Autodesk Fusion 360 part; units mm, degrees
sketch "Sketch1" plane through (0, 0, 0) normal (0, 1, 0) x (1, 0, 0)
  line L0 (0, 0) -> (56, 0)
  line L1 (56, 0) -> (56, -65)
  line L2 (56, -65) -> (0, -65)
  line L3 (0, -65) -> (0, 0)
  dimension "d1" = 56
  dimension "d2" = 65
extrude "Extrude1" add sketch "Sketch1" along normal blind 1
sketch "Sketch2" plane through (0, 1, 0) normal (0, 1, 0) x (-1, 0, 0)
  line L0 (0, 65) -> (-56, 65)
  line L1 (-56, 65) -> (-56, 0)
  line L2 (-56, 0) -> (0, 0)
  line L3 (0, 0) -> (0, 65)
  line L4 (-1.5, 7) -> (-5.5, 7)
  line L5 (-5.5, 7) -> (-5.5, 58)
  line L6 (-5.5, 58) -> (-1.5, 58)
  line L7 (-1.5, 58) -> (-1.5, 7)
  dimension "d5" = 4
  dimension "d6" = 51
  dimension "d7" = 7
  dimension "d8" = 7
  dimension "d9" = 1.5
extrude "Extrude2" add sketch "Sketch2" along normal blind 11 contours L4 L5 L6 L7
sketch "Sketch3" plane through (0, 0, 0) normal (0, -1, 0) x (1, 0, 0)
  line L0 (56, 65) -> (0, 65)
  line L1 (0, 65) -> (0, 0)
  line L2 (0, 0) -> (56, 0)
  line L3 (56, 0) -> (56, 65)
  line L4 (1.5, 7) -> (5.5, 7)
  line L5 (5.5, 7) -> (5.5, 58)
  line L6 (5.5, 58) -> (1.5, 58)
  line L7 (1.5, 58) -> (1.5, 7)
extrude "Extrude3" add sketch "Sketch3" along normal blind 14 contours L4 L5 L6 L7
sketch "Sketch4" plane through (0, 1, 0) normal (0, 1, 0) x (-1, 0, 0)
  line L0 (-1.5, 58) -> (-1.5, 7)
  line L1 (-1.5, 7) -> (-5.5, 7)
  line L2 (-5.5, 7) -> (-5.5, 58)
  line L3 (-5.5, 58) -> (-1.5, 58)
  line L4 (0, 65) -> (-56, 65)
  line L5 (-56, 65) -> (-56, 0)
  line L6 (-56, 0) -> (0, 0)
  line L7 (0, 0) -> (0, 65)
  line L8 (-11.1237, 3.0691) -> (-51.1237, 3.0691)
  line L9 (-51.1237, 3.0691) -> (-51.1237, 63.0691)
  line L10 (-51.1237, 63.0691) -> (-11.1237, 63.0691)
  line L11 (-11.1237, 63.0691) -> (-11.1237, 3.0691)
  dimension "d14" = 40
  dimension "d15" = 60
extrude "Extrude4" add sketch "Sketch4" along normal blind 9 contours L8 L9 L10 L11
For this review, take the finished solid that the model builds, in its own axes (mm). A direction names the side the tool comes from. Coordinates: 2 decimals unless noted, no trailing zeros. Write each loop counter-clockwise with the first axis right and the second up, starting at its lowest first coordinate (ties: lowest second). Pieces come first, ordered by that corner, then holes. Notation, with made-up numbers: (-10.75, 86) - (5.25, 86) arc R14 ccw to (5.25, 96) - close; hole circle Ø4 at (11, -35.5). An arc over 180 degrees is marked (long way). Put each result on its own line as item: value.
1. For pin 1 (4.5 mm diameter, centred on x = 40, y = 3.5, fed in from +Z); pin 2 (3.5 mm diameter, centred on y = 6.5, z = 20, fed in from +X); pin 3 (4.5 mm diameter, centred on y = 5, z = 22, fed in from -X), all flat-tipped, find the tip position at first contact; note any pin that passes through.
Values found:
pin 1: z = 63.07
pin 2: x = 51.12
pin 3: x = 1.5
2. Mouldability with a two-part tool opening along X and no side actions: class faces 5 (the flat face through (5.5, -7, 32)), 6 (the flat face through (1.5, 6, 33)), 7 (the flat face through (11.124, 5, 33)) as released by +X, released by -X, zero draft, split by the parting line, or undercut.
Values found:
face 5: released by +X
face 6: released by -X
face 7: undercut
3. Machinability: for faces 1 (the flat face through (4, -7, 58)), 2 (the flat face through (1.5, -7, 33)), 3 (the flat face through (31, 5, 3.069)), 4 (the flat face through (3, -7, 7)), which of the approach directions +Z, -Z, +X, -X, +Y, -Y give a long, thin tool a straight path to every point of the face, cutting with its end or side? Answer none if there is none.
Values found:
face 1: +Z, +X, -X, -Y
face 2: +Z, -Z, -X, -Y
face 3: -Z, +X, -X, +Y
face 4: -Z, +X, -X, -Y
4. Add section B-B, the plane z = 22. Give the boundary of the cut face in (x, y).
Values found:
outline: (0, 0) - (1.5, 0) - (1.5, -14) - (5.5, -14) - (5.5, 0) - (56, 0) - (56, 1) - (51.12, 1) - (51.12, 10) - (11.12, 10) - (11.12, 1) - (5.5, 1) - (5.5, 12) - (1.5, 12) - (1.5, 1) - (0, 1) - close
5. Add section A-A, the plane y = 4.75. Give the boundary of the cut face in (x, z), then the cut area to 3 significant figures.
Values found:
outline: (1.5, 7) - (5.5, 7) - (5.5, 58) - (1.5, 58) - close; (11.12, 3.07) - (51.12, 3.07) - (51.12, 63.07) - (11.12, 63.07) - close
area: 2,600 mm²
6. Add section C-C, the plane x = 28. Give the boundary of the cut face in (y, z), then the cut area to 3 significant figures.
Values found:
outline: (0, 0) - (1, 0) - (1, 3.07) - (10, 3.07) - (10, 63.07) - (1, 63.07) - (1, 65) - (0, 65) - close
area: 605 mm²
7. Wall thickness on probe 1 along X at (y, z) = (7.5, 31); probe 2 along Y at (x, z) = (47.5, 28); probe 3 along X at (y, z) = (-4.5, 40): over which ranges is each line inside the solid? List them lowest first.
Values found:
probe 1: 1.5 to 5.5, 11.12 to 51.12
probe 2: 0 to 10
probe 3: 1.5 to 5.5
8. Add section D-D, the plane z = 61. Give the boundary of the cut face in (x, y), then the cut area to 3 significant figures.
Values found:
outline: (0, 0) - (56, 0) - (56, 1) - (51.12, 1) - (51.12, 10) - (11.12, 10) - (11.12, 1) - (0, 1) - close
area: 416 mm²
